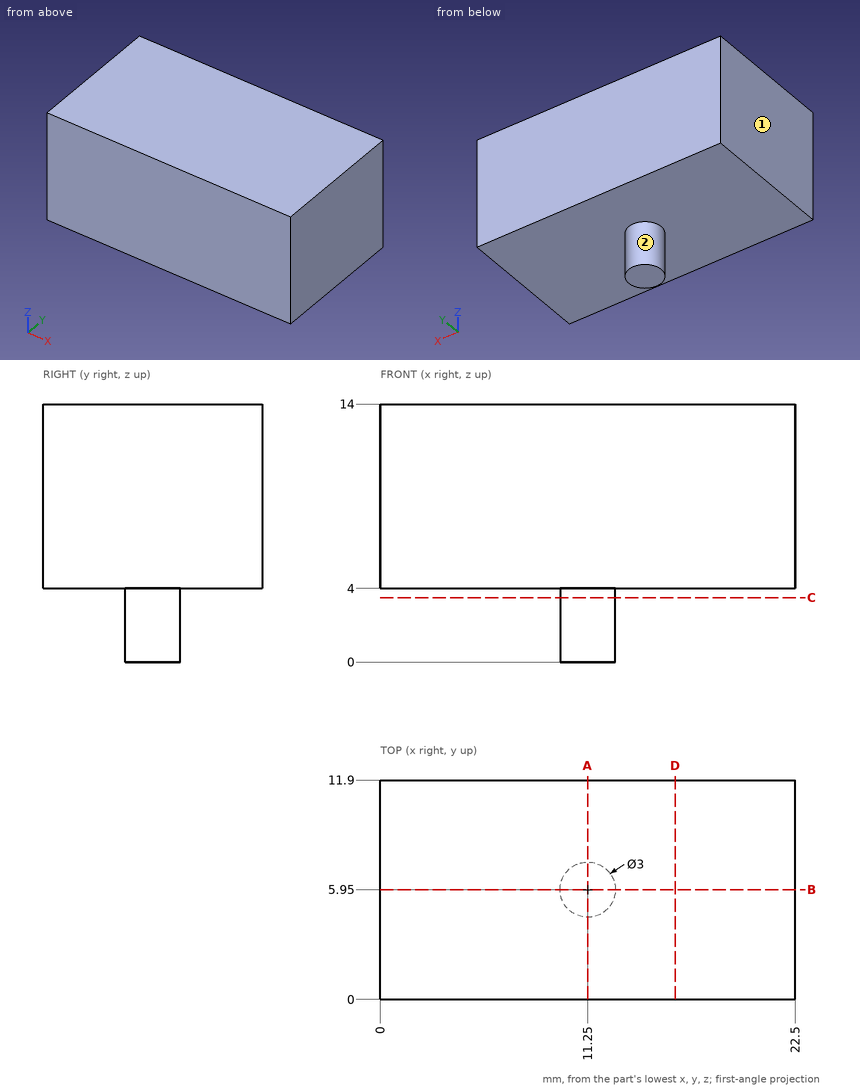
Design review of the part shown in the three views and the two pictorial views. Dimensions are in mm from the part's minimum x, y and z. A direction names the side the tool comes from. Round coordinates to 2 decimals unless told otherwise and drop trailing zeros. Loops run counter-clockwise (first coordinate to the right, second up) from the corner with the lowest first, then second, coordinate; pieces in that order, holes last.
Q1. To check wall thickness, follow line 1 along Z through (x, y) = (6.75, 5.25); line 2 along X through (y, z) = (6.75, 2.25); line 3 along X through (y, z) = (7, 2.25). State the ranges of each line that lie inside material, in increasing order.
Result sheet:
line 1: z = 4 to 14
line 2: x = 9.98 to 12.52
line 3: x = 10.18 to 12.32
Q2. Add section A-A on x = 11.25. Write out the cut boundary in (y, z), plus the area to 3 significant figures.
Result sheet:
outline: (0, 4) - (4.45, 4) - (4.45, 0) - (7.45, 0) - (7.45, 4) - (11.9, 4) - (11.9, 14) - (0, 14) - close
area: 131 mm2
Q3. Machinability: for the marked faces 1 and 2, which of the approach directions +Z, -Z, +X, -X, +Y, -Y give a long, thin tool a straight path to every point of the face, cutting with its end or side? Answer none if there is none.
Result sheet:
face 1: +Z, -Z, -X, +Y, -Y
face 2: -Z
Q4. Add section D-D on x = 16. Write out the cut boundary in (y, z), plus the area to 3 significant figures.
Result sheet:
outline: (0, 4) - (11.9, 4) - (11.9, 14) - (0, 14) - close
area: 119 mm2
Q5. Add section B-B on y = 5.95. Write out the cut boundary in (x, z).
Result sheet:
outline: (0, 4) - (9.75, 4) - (9.75, 0) - (12.75, 0) - (12.75, 4) - (22.5, 4) - (22.5, 14) - (0, 14) - close
Q6. Insertion check: pin 1 Ø3 at (x, y) = (14, 10) entering from -Z. The pin has a flat end and moves straight along its axis. Give the tip position at first contact, or say it passes through.
Result sheet:
pin 1: stops at z = 4
Q7. Add section C-C on z = 3.5. Write out the cut boundary in (x, y).
Result sheet:
outline: circle Ø3 at (11.25, 5.95)
